For this review, use the dimensioned drawing (mm, ordinates from the lowest corner) and the shaded views. A direction names the side the tool comes from. Coordinates: 2 decimals unless noted, no trailing zeros. Write each loop counter-clockwise with the first axis right and the second up, starting at its lowest first coordinate (ties: lowest second). Pieces come first, ordered by that corner, then holes.
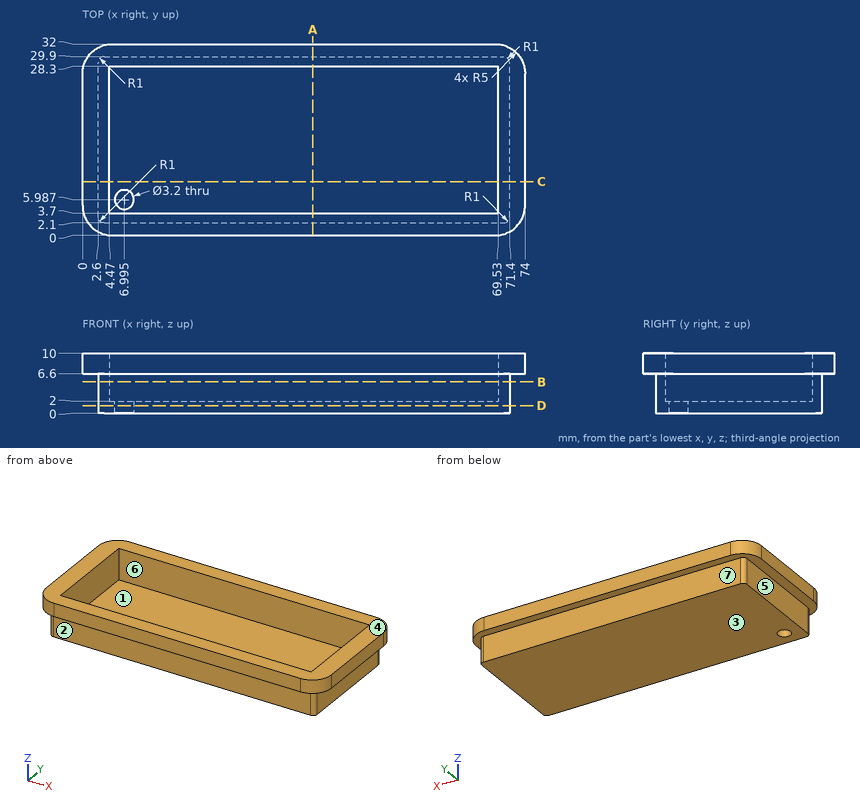
Item 1: Take a section at D-D, the plane z = 1.25. Write out the cut boundary in (x, y) (1 decimal).
Solved:
outline: (2.6, 3.1) arc R1 ccw to (3.6, 2.1) - (70.4, 2.1) arc R1 ccw to (71.4, 3.1) - (71.4, 28.9) arc R1 ccw to (70.4, 29.9) - (3.6, 29.9) arc R1 ccw to (2.6, 28.9) - close; hole circle Ø3.2 at (7, 6)
Item 2: Take a section at A-A, the plane x = 38.5. Write out the cut boundary in (y, z).
Solved:
outline: (0, 6.6) - (2.1, 6.6) - (2.1, 0) - (29.9, 0) - (29.9, 6.6) - (32, 6.6) - (32, 10) - (28.3, 10) - (28.3, 2) - (3.7, 2) - (3.7, 10) - (0, 10) - close
Item 3: Machinability: for the marked faces 4, 5, 6 and 7, which of the approach directions +Z, -Z, +X, -X, +Y, -Y give a long, thin tool a straight path to every point of the face, cutting with its end or side? Answer none if there is none.
Solved:
face 4: +Z, +X, -X, +Y, -Y
face 5: -Z, -X, +Y, -Y
face 6: +Z
face 7: -Z, +X, -X, +Y
Item 4: For pin 1 (2 mm diameter, centred on x = 56, z = 4, fed in from +Y); pin 2 (5.5 mm diameter, centred on y = 20.5, z = 3, fed in from +X); pin 3 (4 mm diameter, centred on x = 7, y = 5.99, fed in from +Z), all flat-tipped, find the tip position at first contact; note any pin that passes through.
Solved:
pin 1: stops at y = 29.9
pin 2: stops at x = 71.4
pin 3: stops at z = 2
Item 5: Take a section at C-C, the plane y = 9. Write out the cut boundary in (x, z), plus the area to 3 significant figures.
Solved:
outline: (0, 6.6) - (2.6, 6.6) - (2.6, 0) - (71.4, 0) - (71.4, 6.6) - (74, 6.6) - (74, 10) - (69.53, 10) - (69.53, 2) - (4.47, 2) - (4.47, 10) - (0, 10) - close
area: 185 mm2
Item 6: Mouldability with a two-part tool opening along Y and no side actions: class the marked faces 1, 2 and 3 as pulls with the +Y half, pulls with the -Y half, needs draft (parallel to the pull), parting line crosses it, or undercut.
Solved:
face 1: undercut
face 2: pulls with the -Y half
face 3: needs draft
Item 7: Take a section at B-B, the plane z = 5.25. Write out the cut boundary in (x, y).
Solved:
outline: (2.6, 3.1) arc R1 ccw to (3.6, 2.1) - (70.4, 2.1) arc R1 ccw to (71.4, 3.1) - (71.4, 28.9) arc R1 ccw to (70.4, 29.9) - (3.6, 29.9) arc R1 ccw to (2.6, 28.9) - close; hole (4.47, 3.7) - (69.53, 3.7) - (69.53, 28.3) - (4.47, 28.3) - close
Item 8: To check wall thickness, follow line 1 along X through (y, z) = (4.5, 3.75); line 2 along Y through (x, z) = (37, 3.75); line 3 along Y through (x, z) = (41, 9.75). State the ranges of each line that lie inside material, in increasing order.
Solved:
line 1: x = 2.6 to 4.47, 69.53 to 71.4
line 2: y = 2.1 to 3.7, 28.3 to 29.9
line 3: y = 0 to 3.7, 28.3 to 32
